Can you work these out from the model? Positions are in its coordinate system, mm. A direction names the side the tool comes from. Give positions to 0.01 mm unless a question says otherwise; leave off trailing zeros. Loops run counter-clockwise (first coordinate to the right, second up) from the corner with the lowest first, then second, coordinate; pieces in that order, holes last. Notation, with made-up numbers: (-4.5, 45) - (50.5, 45) arc R36 cw to (50.5, 84) - close; hole circle Ø3 at (-31.75, 41). An arc over 180 degrees is marked (long way). Answer as a JSON object with one key per item and string values. Group by question number.
Item 1: Please list where these lines run through material, in increasing order: L1, parallel to Z at x = 17, y = 7.5; L2, parallel to Y at x = 23.25, z = 135; L3, parallel to X at y = 11.5, z = 146.
Item 2: Thinking about a two-plate mould opening in Z: for faces 4 (the cylindrical face through (20.153, 1.782, 145.234)), 5 (the flat face through (17, 8, -10)), 6 (the flat face through (17, 15, 71)), which applies, pulls with the +Z half, pulls with the -Z half, needs draft (parallel to the pull), parting line crosses it, or undercut?
Item 3: Suppose I cut it at A-A on x = 17. Write out the boundary of the cut face in (y, z).
Item 4: Suppose I cut it at B-B on z = 18. Write out the boundary of the cut face in (x, y).
Item 5: Will these pins go through, and if not, where does the flat tip stop? pin 1 (6.5 mm diameter, centred on y = 6.5, z = 88, fed in from +X); pin 2 (1 mm diameter, centred on y = 8.5, z = 132, fed in from +X); pin 3 (2.5 mm diameter, centred on x = 22, z = 146, fed in from -Y).
Item 6: Which directions (+Z, -Z, +X, -X, +Y, -Y) give clear straight access to the entire face, cutting with the end or side of a thin tool? Please do faces 1 (the flat face through (20, 7, 69)), 2 (the flat face through (17, 7, 150)), 3 (the flat face through (14, 7, 69)).
Item 7: Suppose I cut it at C-C on y = 6. Write out the boundary of the cut face in (x, z), and give its area (3 significant figures).
Autodesk Fusion 360 part; units mm, degrees
sketch "Sketch1" plane through (0, 0, 0) normal (1, 0, 0) x (0, 0, -1)
  line L0 (-150, 0) -> (-150, 10)
  line L1 (-150, 10) -> (0, 10)
  line L2 (0, 10) -> (0, 0)
  line L3 (-150, 10) -> (-140, 10)
  line L4 (-140, 10) -> (-140, 0)
  line L5 (-140, 0) -> (-150, 0)
  line L6 (-150, 0) -> (-150, 10)
  line L7 (0, 0) -> (-10, 0)
  line L8 (-10, 0) -> (-10, 10)
  line L9 (-10, 10) -> (0, 10)
  line L10 (0, 10) -> (0, 0)
  line L11 (-2.5, 0) -> (-12.5, 0)
  line L12 (-12.5, 10) -> (-2.5, 10)
  line L13 (-150, 0) -> (-147.5, 0)
  line L14 (0, 0) -> (-147.5, 0)
  dimension "d2" = 10
  dimension "d3" = 130
  dimension "d4" = 10
  dimension "d9" = 10
  dimension "d11" = 10
extrude "Extrude1" add sketch "Sketch1" along normal blind 15
extrude "Extrude4" add 1 faces at (15, 6.6667, 100) along direction (1, 0, 0) blind 10
extrude "Extrude5" add 1 faces at (16.6667, 10, 50) along direction (0, 1, 0) blind 5
sketch "Sketch2" plane through (0, 0, 0) normal (0, 0, -1) x (-1, 0, 0)
  line L0 (0, 15) -> (-25, 15)
  line L1 (-25, 15) -> (-25, 0)
  line L2 (-25, 0) -> (0, 0)
  line L3 (-25, 0) -> (-25, 3)
  line L4 (-25, 15) -> (-25, 12)
  line L5 (-23.5, 10.5) -> (-25, 12)
  line L6 (-23.5, 4.5) -> (-25, 3)
  line L7 (-23.5, 4.5) -> (-23.5, 2.5)
  line L8 (-23.5, 12.5) -> (-22, 12.5)
  line L9 (-23.5, 2.5) -> (-22, 2.5)
  line L10 (-22, 2.5) -> (-20, 4.5)
  line L11 (-20, 4.5) -> (-20, 10.5)
  line L12 (-20, 10.5) -> (-22, 12.5)
  line L13 (-23.5, 2.5) -> (-23.5, 4.5)
  line L14 (-23.5, 10.5) -> (-23.5, 12.5)
  line L15 (-20, 4.5) -> (-14, 4.5)
  line L16 (-14, 4.5) -> (-14, 10.5)
  line L17 (-14, 10.5) -> (-20, 10.5)
  line L18 (-20, 10.5) -> (-20, 4.5)
  line L19 (-17, 4.5) -> (-17, 10.5)
  line L20 (-14, 7.5) -> (-20, 7.5)
  line L21 (-10.5, 4.5) -> (-9, 3)
  line L22 (-10.5, 2.5) -> (-10.5, 4.5)
  line L23 (-10.5, 2.5) -> (-12, 2.5)
  line L24 (-12, 2.5) -> (-14, 4.5)
  line L25 (-14, 4.5) -> (-14, 10.5)
  line L26 (-14, 10.5) -> (-12, 12.5)
  line L27 (-10.5, 12.5) -> (-12, 12.5)
  line L28 (-10.5, 10.5) -> (-10.5, 12.5)
  line L29 (-10.5, 10.5) -> (-9, 12)
  line L30 (-9, 3) -> (-9, 12)
  line L31 (-9, 0) -> (-25, 0)
  line L32 (-25, 0) -> (-25, 15)
  line L33 (-25, 15) -> (-9, 15)
  line L34 (-9, 15) -> (-9, 0)
  line L35 (0, 0) -> (-15, 0)
  line L36 (-15, 0) -> (-15, 15)
  line L37 (-15, 15) -> (0, 15)
  line L38 (0, 15) -> (0, 0)
  line L39 (0, 0) -> (0, 15)
  dimension "d22" = 3
  dimension "d23" = 3
  dimension "d24" = 6
  dimension "d27" = 10
  dimension "d28" = 6
  dimension "d29" = 135
  dimension "d30" = 135
  dimension "d31" = 45
  dimension "d32" = 45.001
  dimension "d33" = 1.5
  dimension "d34" = 1.5
  dimension "d35" = 2.1213
  dimension "d37" = 2
  dimension "d38" = 6
  dimension "d39" = 6
  dimension "d40" = 16
  dimension "d45" = 15
  dimension "d48" = 15
extrude "Extrude6" cut sketch "Sketch2" against normal blind 185 contours L16 L21 L22 L23 L24 L25 L26 L27 L28 L29 L30 L34 | L1 L5 L6 L7 L8 L9 L10 L11 L12 L13 L14 L18 L32
extrude "Extrude8" add sketch "Sketch2" along normal blind 10 contours L0 L17 L26 L27 L28 L29 L33 L34 L36 L37 | L0 L1 L4 L5 L8 L12 L14 L17 L32 L33 L36 | L2 L15 L21 L22 L23 L24 L31 L34 L35 L36 | L17 L19 L20 L36 | L16 L17 L20 L25 L36 | L1 L2 L3 L6 L7 L9 L10 L13 L15 L31 L32 L36 | L11 L17 L18 L19 L20 | L15 L19 L20 L36 | L15 L16 L20 L25 L36 | L11 L15 L18 L19 L20
extrude "Extrude9" cut 1 faces at (3, 6, 0) along direction (0, 0, 1) blind 240
sketch "Sketch3" plane through (0, 0, 0) normal (0, -1, 0) x (1, 0, 0)
  line L0 (9, 150) -> (9, -10)
  line L1 (9, -10) -> (25, -10)
  line L2 (25, -10) -> (25, 150)
  line L3 (25, 150) -> (9, 150)
  line L4 (25, 150) -> (25, 145)
  line L5 (25, 145) -> (9, 145)
  line L6 (9, 145) -> (9, -5)
  line L7 (9, -5) -> (25, -5)
  line L8 (25, -5) -> (25, 145)
  line L9 (25, 145) -> (9, 145)
  line L10 (9, 145) -> (9, 135)
  line L11 (9, 135) -> (25, 135)
  line L12 (25, 135) -> (25, 145)
  line L13 (9, -5) -> (25, -5)
  line L14 (25, -5) -> (25, 5)
  line L15 (25, 5) -> (9, 5)
  line L16 (9, 5) -> (9, -5)
  circle A0 centre (17, -0.0404) radius 2
  circle A1 centre (17, 140) radius 2
  dimension "d51" = 16
  dimension "d52" = 150
  dimension "d53" = 5
  dimension "d54" = 10
  dimension "d55" = 130
  dimension "d56" = 16
  dimension "d63" = 4
  dimension "d64" = 4
  dimension "d65" = 140.0404
extrude "Extrude10" cut sketch "Sketch3" against normal blind 50 contours A0 | A1
sketch "Sketch4" plane through (0, 15, 0) normal (0, 1, 0) x (-1, 0, 0)
  circle A0 centre (-17, 140) radius 2
  circle A1 centre (-17, -0.0404) radius 2
  line L0 (-9, -10) -> (-9, 150)
  line L1 (-9, 150) -> (-25, 150)
  line L2 (-25, 150) -> (-25, -10)
  line L3 (-25, -10) -> (-9, -10)
  circle A2 centre (-12, 146) radius 2
  circle A3 centre (-22, 146) radius 2
  dimension "d66" = 4
  dimension "d68" = 4
  dimension "d69" = 3
  dimension "d70" = 3
  dimension "d71" = 4
  dimension "d72" = 4
extrude "Extrude11" cut sketch "Sketch4" against normal blind 24 contours A2 | A3
Worked out:
{
 "1": {"L1": "z = -10 to -2.04, 1.96 to 138, 142 to 150", "L2": "y = 0 to 2.5, 12.5 to 15", "L3": "x = 9.5 to 10, 14 to 20, 24 to 24.5"},
 "2": {"face 4": "undercut", "face 5": "pulls with the -Z half", "face 6": "needs draft"},
 "3": {"outline": "(0, -10) - (15, -10) - (15, -2.04) - (0, -2.04) - close; (0, 1.96) - (15, 1.96) - (15, 138) - (0, 138) - close; (0, 142) - (15, 142) - (15, 150) - (0, 150) - close"},
 "4": {"outline": "(9, 0) - (25, 0) - (25, 3) - (23.5, 4.5) - (23.5, 2.5) - (22, 2.5) - (20, 4.5) - (20, 10.5) - (22, 12.5) - (23.5, 12.5) - (23.5, 10.5) - (25, 12) - (25, 15) - (9, 15) - (9, 12) - (10.5, 10.5) - (10.5, 12.5) - (12, 12.5) - (14, 10.5) - (14, 4.5) - (12, 2.5) - (10.5, 2.5) - (10.5, 4.5) - (9, 3) - close"},
 "5": {"pin 1": "stops at x = 24.75", "pin 2": "stops at x = 20", "pin 3": "passes through"},
 "6": {"face 1": "+Z, -Z, +X", "face 2": "+Z, +X, -X, +Y, -Y", "face 3": "+Z, -Z, -X"},
 "7": {"outline": "(14, -10) - (20, -10) - (20, 150) - (14, 150) - close; hole circle Ø4 at (17, -0.04); hole circle Ø4 at (17, 140)", "area": "935 mm2"}
}
